Read the model definition and answer for the solid it produces. Units are mm, in the model's axes. Face numbers are marked on the shaded views. A direction names the side the tool comes from. Round coordinates to 2 decimals unless told otherwise and drop trailing zeros. Loops run counter-clockwise (first coordinate to the right, second up) from the corner with the lowest first, then second, coordinate; pieces in that order, holes last. Notation, with made-up numbers: (1, 3) - (57, 3) arc R20 ccw to (57, 32) - close; hole circle Ø9 at (-28, -14). An arc over 180 degrees is marked (long way). Answer as CSV lines item,"result".
```python
from build123d import *

# Parameters (mm, degrees)
BOSS_EXTRUDE5_DEPTH = 95
FILLET16_R          = 15
FILLET17_R          = 15
FILLET18_R          = 15
FILLET19_R          = 15
FILLET21_R          = 5
FILLET22_R          = 5
FILLET23_R          = 5
FILLET24_R          = 5
FILLET25_R          = 5
FILLET26_R          = 5
FILLET28_R          = 5
FILLET29_R          = 5
FILLET30_R          = 5
FILLET31_R          = 5


with BuildPart() as part:
    # Sketch2 → Boss-Extrude5 (new body)
    with BuildSketch(Plane(origin=(0, 0, 0), x_dir=(1, 0, 0), z_dir=(0, 1, 0))):
        Polygon((-11.5, 10.5), (11.453517933, 10.5), (23.299541019, 15.223771191), (26.5, 15.223771191), (26.5, 16.5), (36.5, 16.5), (36.5, 13.259608353), (16.5, 6.5), (16.5, -6.5), (-16.5, -6.5), (-16.5, 6.5), (-37.988921901, 13.259608353), (-37.988921901, 16.5), (-27.988921901, 16.5), (-27.970531324, 16.5), (-27.970531324, 16.440454109), (-27.970531324, 15.223771191), (-24.481649041, 15.223771191), align=None)
    extrude(amount=BOSS_EXTRUDE5_DEPTH)

    # Fillet16
    # the kernel refuses this fillet: 15 mm, written as the material it takes off along each edge
    with BuildSketch(Plane(origin=(36.5, -20.136972883, -13.259608353), x_dir=(-0.9473542933434234, 0, 0.3201871997500573), z_dir=(0, 1, 0))) as fillet16_piece_1:
        with BuildLine():
            CenterArc((8.054789153, -15), FILLET16_R, 90, 37.311981857)
            Line((-1.037531927, -3.069798938), (-1.219378349, -2.831194917))
            ThreePointArc((-1.219378349, -2.831194917), (-0.802972252, -1.438843309), (-0.284206288, 0.09605616))
            Line((-0.284206288, 0.09605616), (0, 0.3))
            Line((0, 0.3), (8.054789153, 0.3))
            Line((8.054789153, 0.3), (8.054789153, 0))
        make_face()
    extrude(amount=135.273945765, mode=Mode.SUBTRACT)

    # Fillet17
    # the kernel refuses this fillet: 15 mm, written as the material it takes off along each edge
    with BuildSketch(Plane(origin=(-37.988921901, -20.369568994, -13.259608353), x_dir=(0, 0, -1), z_dir=(0, 1, 0))) as fillet17_piece_1:
        with BuildLine():
            CenterArc((11.863879582, -12.273363672), FILLET17_R, 125.092573115, 37.445808138)
            Line((-2.444893018, -7.772360819), (-2.73106847, -7.682340761))
            Line((-2.73106847, -7.682340761), (-0.286175452, 0.090020057))
            Line((-0.286175452, 0.090020057), (0, 0.3))
            ThreePointArc((0, 0.3), (1.620195823, 0.3), (3.067921888, 0.245467273))
            Line((3.067921888, 0.245467273), (3.240391647, 0))
        make_face()
    extrude(amount=135.739137989, mode=Mode.SUBTRACT)

    # Fillet18
    fillet18_edges = [part.edges().sort_by_distance(p)[0] for p in [
        (23.299541019, 47.5, -15.223771191),
    ]]
    fillet(fillet18_edges, radius=FILLET18_R)

    # Fillet19
    fillet19_edges = [part.edges().sort_by_distance(p)[0] for p in [
        (-24.481649041, 47.5, -15.223771191),
    ]]
    fillet(fillet19_edges, radius=FILLET19_R)

    # Fillet21
    # the kernel refuses this fillet: 5 mm, written as the material it takes off along each edge
    with BuildSketch(Plane(origin=(26.5, -8.341735474, -16.5), x_dir=(0, 0, 1), z_dir=(0, 1, 0))) as fillet21_piece_1:
        with BuildLine():
            CenterArc((5, 3.33669419), FILLET21_R, 180, 41.862005804)
            Line((0, 3.33669419), (-0.1, 3.33669419))
            Line((-0.1, 3.33669419), (-0.1, 0))
            Line((-0.1, 0), (0, -0.1))
            ThreePointArc((0, -0.1), (0.638114404, -0.1), (1.201753385, -0.066733884))
            Line((1.201753385, -0.066733884), (1.276228809, 0))
        make_face()
    extrude(amount=111.683470949, mode=Mode.SUBTRACT)

    # Fillet22
    # the kernel refuses this fillet: 5 mm, written as the material it takes off along each edge
    with BuildSketch(Plane(origin=(-27.970531324, -8.341735474, -16.5), x_dir=(0, 0, 1), z_dir=(0, 1, 0))) as fillet22_piece_1:
        with BuildLine():
            CenterArc((5, -3.33669419), FILLET22_R, 138.137994196, 41.862005804)
            Line((0, -3.33669419), (-0.1, -3.33669419))
            Line((-0.1, -3.33669419), (-0.1, 0))
            Line((-0.1, 0), (0, 0.1))
            ThreePointArc((0, 0.1), (0.638114404, 0.1), (1.201753385, 0.066733884))
            Line((1.201753385, 0.066733884), (1.276228809, 0))
        make_face()
    extrude(amount=111.683470949, mode=Mode.SUBTRACT)

    # Fillet23
    # the kernel refuses this fillet: 5 mm, written as the material it takes off along each edge
    with BuildSketch(Plane(origin=(-4.576022833, 0, -2.749164289), x_dir=(0.3000668568991913, 0, -0.9539181733202489), z_dir=(-0.9539181733202489, 0, -0.3000668568991913))) as fillet23_piece_1_section:
        with BuildLine():
            CenterArc((FILLET23_R, -FILLET23_R), FILLET23_R, 90, 90)
            Line((0, -FILLET23_R), (-FILLET23_R * 0.02, -FILLET23_R))
            Line((-FILLET23_R * 0.02, -FILLET23_R), (-FILLET23_R * 0.02, FILLET23_R * 0.02))
            Line((-FILLET23_R * 0.02, FILLET23_R * 0.02), (FILLET23_R, FILLET23_R * 0.02))
            Line((FILLET23_R, FILLET23_R * 0.02), (FILLET23_R, 0))
        make_face()
    fillet23_piece_1 = extrude(amount=26.879179961, mode=Mode.PRIVATE)
    fillet23_piece_1 = split(fillet23_piece_1, bisect_by=Plane(origin=(-16.5, 1.14737311, -9.7645004), z_dir=(-1, 0, 0)), keep=Keep.TOP, mode=Mode.PRIVATE)
    add(fillet23_piece_1, mode=Mode.SUBTRACT)
    with BuildSketch(Plane(origin=(-25.715558229, 0, -25.123487935), x_dir=(-0.3000668568991974, 0, 0.9539181733202469), z_dir=(0.9539181733202469, 0, 0.3000668568991974))) as fillet23_piece_2_section:
        with BuildLine():
            CenterArc((15 - FILLET23_R, -FILLET23_R), FILLET23_R, 0, 90)
            Line((15, -FILLET23_R), (15 + FILLET23_R * 0.02, -FILLET23_R))
            Line((15 + FILLET23_R * 0.02, -FILLET23_R), (15 + FILLET23_R * 0.02, FILLET23_R * 0.02))
            Line((15 + FILLET23_R * 0.02, FILLET23_R * 0.02), (15 - FILLET23_R, FILLET23_R * 0.02))
            Line((15 - FILLET23_R, FILLET23_R * 0.02), (15 - FILLET23_R, 0))
        make_face()
    fillet23_piece_2 = revolve(axis=Axis((-25.715558229, 0, -25.123487935), (0, -1, 0)), revolution_arc=85.195610564, mode=Mode.PRIVATE)
    fillet23_piece_2 = split(fillet23_piece_2, bisect_by=Plane(origin=(-33.617328681, 1.250053693, -16.5), z_dir=(0, 0, 1)), keep=Keep.TOP, mode=Mode.PRIVATE)
    add(fillet23_piece_2, mode=Mode.SUBTRACT)

    # Fillet24
    fillet24_edges = [part.edges().sort_by_distance(p)[0] for p in [
        (22.684630457, 0, -8.590283985),
        (33.162574695, 0, -12.963578877),
    ]]
    fillet(fillet24_edges, radius=FILLET24_R)

    # Fillet25
    fillet25_edges = [part.edges().sort_by_distance(p)[0] for p in [
        (33.162574695, 95, -12.963578877),
        (22.684630457, 95, -8.590283985),
    ]]
    fillet(fillet25_edges, radius=FILLET25_R)

    # Fillet26
    # the kernel refuses this fillet: 5 mm, written as the material it takes off along each edge
    with BuildSketch(Plane(origin=(-25.715558229, 95, -25.123487935), x_dir=(-0.3000668568991974, 0, 0.9539181733202469), z_dir=(0.9539181733202469, 0, 0.3000668568991974))) as fillet26_piece_1:
        with BuildLine():
            CenterArc((15 - FILLET26_R, FILLET26_R), FILLET26_R, 270, 90)
            Line((15, FILLET26_R), (15, 0))
            Line((15, 0), (15 - FILLET26_R, 0))
        make_face()
    revolve(axis=Axis((-25.715558229, 95, -25.123487935), (0, -1, 0)), revolution_arc=85.195610564, mode=Mode.SUBTRACT)
    with BuildSketch(Plane(origin=(-4.576022833, 95, -2.749164289), x_dir=(0.3000668568991913, 0, -0.9539181733202489), z_dir=(-0.9539181733202489, 0, -0.3000668568991913))) as fillet26_piece_2_section:
        with BuildLine():
            CenterArc((FILLET26_R, FILLET26_R), FILLET26_R, 180, 90)
            Line((0, FILLET26_R), (0, 0))
            Line((0, 0), (FILLET26_R, 0))
        make_face()
    fillet26_piece_2 = extrude(amount=26.879179961, mode=Mode.PRIVATE)
    fillet26_piece_2 = split(fillet26_piece_2, bisect_by=Plane(origin=(-16.5, 93.85262689, -9.7645004), z_dir=(-1, 0, 0)), keep=Keep.TOP, mode=Mode.PRIVATE)
    add(fillet26_piece_2, mode=Mode.SUBTRACT)

    # Fillet28
    fillet28_edges = [part.edges().sort_by_distance(p)[0] for p in [
        (16.5, 0, -2.638928242),
    ]]
    fillet(fillet28_edges, radius=FILLET28_R)

    # Fillet29
    fillet29_edges = [part.edges().sort_by_distance(p)[0] for p in [
        (-16.5, 0, -2.620769863),
    ]]
    fillet(fillet29_edges, radius=FILLET29_R)

    # Fillet30
    fillet30_edges = [part.edges().sort_by_distance(p)[0] for p in [
        (-16.5, 95, -2.620769863),
    ]]
    fillet(fillet30_edges, radius=FILLET30_R)

    # Fillet31
    fillet31_edges = [part.edges().sort_by_distance(p)[0] for p in [
        (16.5, 95, -2.638928242),
    ]]
    fillet(fillet31_edges, radius=FILLET31_R)


solid = part.part
```
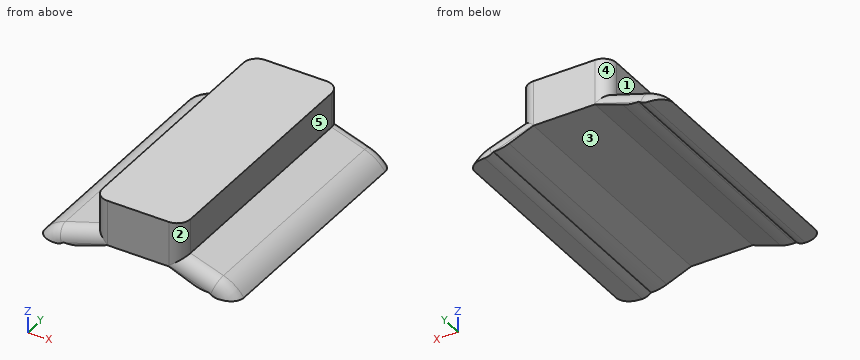
1) Each of these flat-tipped pins is pushed along its axis until it touches: P1, Ø3, axis at y = 56.5, z = -11, coming from the +X side; P2, Ø10.5, axis at y = 66, z = 1.5, coming from the +X side; P3, Ø7, axis at x = -4.5, y = 39, coming from the -Z side; P4, Ø3, axis at x = -30.5, y = 17.5, coming from the -Z side. Where does it stop, or does it pass through?
Entries:
P1,"stops at x = 32.52"
P2,"stops at x = 16.5"
P3,"stops at z = -10.5"
P4,"stops at z = -16.5"
2) A cutting plane is placed at A-A, the plane z = 3. Determine the outline of the cut face in (x, y), plus the area to 3 significant figures.
Entries:
outline,"(-16.5, 5) arc R5 ccw to (-11.5, 0) - (11.5, 0) arc R5 ccw to (16.5, 5) - (16.5, 90) arc R5 ccw to (11.5, 95) - (-11.5, 95) arc R5 ccw to (-16.5, 90) - close"
area,"3,110 mm^2"
3) A cutting plane is placed at C-C, the plane x = -7. Determine the outline of the cut face in (y, z), plus the area to 4 significant figures.
Entries:
outline,"(0, -10.5) - (95, -10.5) - (95, 6.5) - (0, 6.5) - close"
area,"1,615 mm^2"
4) A tool of negligible diameter and unlimited length cuts with its end or side. For the marked faces 1, 2, 3, 4 and 5, from which of +Z, -Z, +X, -X, +Y, -Y can it reach the whole face along a straight path? Write none if from no direction.
Entries:
face 1,"+Z, -X, +Y, -Y"
face 2,"+Z, +X, -Y"
face 3,"-Z, +Y, -Y"
face 4,"+Z, -X, +Y"
face 5,"+Z, +X, +Y, -Y"
5) A cutting plane is placed at B-B, the plane y = 16. Determine the outline of the cut face in (x, z).
Entries:
outline,"(-37.99, -16.5) - (-31.31, -16.5) arc R5 ccw to (-27.97, -15.22) - (-27.13, -15.22) arc R15 ccw to (-22, -14.32) - (-11.5, -10.5) - (11.45, -10.5) - (20.62, -14.16) arc R15 ccw to (26.18, -15.22) - (26.5, -15.22) arc R5 ccw to (29.84, -16.5) - (36.5, -16.5) arc R15 ccw to (28.87, -10.68) - (16.5, -6.5) - (16.5, 6.5) - (-16.5, 6.5) - (-16.5, -6.5) - (-30.22, -10.81) arc R15 ccw to start"
6) Find the intervals of material crossed by line 1 (Z direction, x = 8, y = 10); line 2 (X direction, y = 70.5, z = 4); line 3 (Z direction, x = -34, y = 26.5), in increasing order.
Entries:
line 1,"z = -10.5 to 6.5"
line 2,"x = -16.5 to 16.5"
line 3,"z = -16.5 to -12.62"
